Here's how the part is built. I have some questions about the finished solid (model axes, mm). Face numbers are marked on the shaded views. A direction names the side the tool comes from. Coordinates: 2 decimals unless noted, no trailing zeros. Order: outer loops, then holes, each group sorted by start corner. A loop starts at its lowest first (then second) coordinate and runs counter-clockwise, first axis right, second up. Notation, with made-up numbers: (71.5, -31) - (104.5, -31) arc R18 ccw to (104.5, -25) - close; hole circle Ø9 at (-16, 15.25). An arc over 180 degrees is marked (long way). Answer as CSV lines item,"result". Start each with the question number.
Item 1: Imagine slicing it at D-D on y = -2.5. List the corners of the cut face in (x, z) for me, and give its area (3 significant figures).
Item 2: We'd pull the mould along Y, two halves only. Please class the marked faces 1, 2 and 3: pulls with the +Y half, pulls with the -Y half, needs draft (parallel to the pull), parting line crosses it, or undercut.
Item 3: On a 3-axis mill with a long thin cutter (end or side, diameter ignored), from which of +Z, -Z, +X, -X, +Y, -Y can I reach the whole of each face in a straight line? I mean the marked faces 4, 5, 6 and 7. Say none if no direction works.
Item 4: I'm going to push flat-ended pins straight in: pin 1 (0.9 mm diameter, centred on y = 5.5, z = 2, fed in from +X); pin 2 (1.5 mm diameter, centred on y = 4, z = 1.5, fed in from -X); pin 3 (1.5 mm diameter, centred on x = -5.5, z = 1, fed in from -Y); pin 4 (4 mm diameter, centred on x = 2.5, y = 2.5, fed in from -Z). Where does each tip first touch, or does it pass through?
Item 5: Imagine slicing it at A-A on x = 5.5. List the corners of the cut face in (y, z) for me, and give its area (3 significant figures).
Item 6: I need wall thicknesses on line 1 (Y direction, x = -6, z = 2.5); line 2 (X direction, y = -0.25, z = 0.8); line 3 (Y direction, x = -3.5, z = 1.1). Which ranges of each line are inside material? Lowest first, please.
Item 7: Imagine slicing it at C-C on x = -5.5. List the corners of the cut face in (y, z) for me, and give its area (3 significant figures).
Item 8: Imagine slicing it at B-B on z = 0.25. List the corners of the cut face in (x, y) for me (3 decimals), and give its area (3 significant figures).
from build123d import *

# Parameters (mm, degrees)
SKETCH1_W           = 10.5
SKETCH1_H           = 22
BOSS_EXTRUDE1_DEPTH = 3
SKETCH2_W           = 6.75
SKETCH2_H           = 3
BOSS_EXTRUDE2_DEPTH = 3
SKETCH3_W           = 3
SKETCH3_H           = 3
BOSS_EXTRUDE3_DEPTH = 3
SKETCH4_W           = 2
SKETCH4_H           = 1.5
CUT_EXTRUDE1_DEPTH  = 3
SKETCH5_W           = 2
SKETCH5_H           = 10.5
CUT_EXTRUDE2_DEPTH  = 3
CHAMFER1_SIZE       = 0.25
CHAMFER2_SIZE       = 0.25
SKETCH6_W           = 3
SKETCH6_H           = 5
CUT_EXTRUDE3_DEPTH  = 0.5


with BuildPart() as part:
    # Sketch1 → Boss-Extrude1 (new body)
    with BuildSketch(Plane.XY):
        with Locations((1.5, 0)):
            Rectangle(SKETCH1_W, SKETCH1_H)
    extrude(amount=BOSS_EXTRUDE1_DEPTH)

    # Sketch2 → Boss-Extrude2 (add)
    with BuildSketch(Plane.XZ.offset(11)):
        with Locations((3, 1.5)):
            Rectangle(SKETCH2_W, SKETCH2_H)
    extrude(amount=BOSS_EXTRUDE2_DEPTH)

    # Sketch3 → Boss-Extrude3 (add)
    with BuildSketch(Plane.ZY.offset(3.75)):
        with Locations((1.5, -6.5)):
            Rectangle(SKETCH3_W, SKETCH3_H)
        with Locations((1.5, 6.5)):
            Rectangle(SKETCH3_W, SKETCH3_H)
    extrude(amount=BOSS_EXTRUDE3_DEPTH)

    # Sketch4 → Cut-Extrude1 (cut)
    with BuildSketch(Plane.XY.offset(3)):
        with Locations((5.75, -5.25)):
            Rectangle(SKETCH4_W, SKETCH4_H)
    extrude(amount=-CUT_EXTRUDE1_DEPTH, mode=Mode.SUBTRACT)

    # Sketch5 → Cut-Extrude2 (cut)
    with BuildSketch(Plane.XY.offset(3)):
        with Locations((5.75, 5.75)):
            Rectangle(SKETCH5_W, SKETCH5_H)
    extrude(amount=-CUT_EXTRUDE2_DEPTH, mode=Mode.SUBTRACT)

    # Chamfer1
    chamfer1_edges = [part.edges().sort_by_distance(p)[0] for p in [
        (4.75, -4.5, 1.5),
    ]]
    chamfer(chamfer1_edges, length=CHAMFER1_SIZE)

    # Chamfer2
    chamfer2_edges = [part.edges().sort_by_distance(p)[0] for p in [
        (4.75, -6, 1.5),
    ]]
    chamfer(chamfer2_edges, length=CHAMFER2_SIZE)

    # Sketch6 → Cut-Extrude3 (cut)
    with BuildSketch(Plane(origin=(6.75, 0, 0), x_dir=(0, 0, -1), z_dir=(1, 0, 0))):
        with Locations((-1.5, -2)):
            Rectangle(SKETCH6_W, SKETCH6_H)
    extrude(amount=-CUT_EXTRUDE3_DEPTH, mode=Mode.SUBTRACT)


solid = part.part
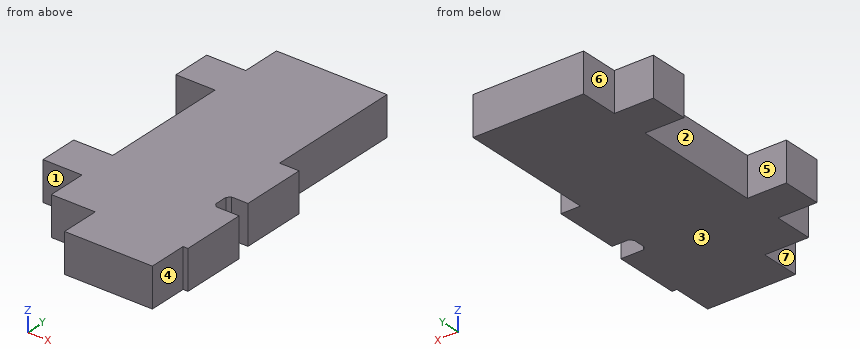
Responses:
1,outline,"(-3.75, 0) - (6.25, 0) - (6.25, 3) - (-3.75, 3) - close"
1,area,"30.0 mm^2"
2,face 1,"pulls with the -Y half"
2,face 2,"undercut"
2,face 3,"needs draft"
3,face 4,"+Z, -Z, +X, -Y"
3,face 5,"+Z, -Z, -X"
3,face 6,"+Z, -Z, -X, +Y"
3,face 7,"+Z, -Z, -X, -Y"
4,pin 1,"stops at x = 4.75"
4,pin 2,"stops at x = -3.75"
4,pin 3,"stops at y = -8"
4,pin 4,"stops at z = 0"
5,outline,"(-14, 0) - (-6, 0) - (-6, 3) - (-14, 3) - close; (-4.5, 0) - (0.5, 0) - (0.5, 3) - (-4.5, 3) - close"
5,area,"39.0 mm^2"
6,line 1,"y = -8 to -5, 5 to 8"
6,line 2,"x = -3.75 to 6.25"
6,line 3,"y = -11 to 11"
7,outline,"(-8, 0) - (-5, 0) - (-5, 3) - (-8, 3) - close; (5, 0) - (8, 0) - (8, 3) - (5, 3) - close"
7,area,"18.0 mm^2"
8,outline,"(-6.75, -8) - (-3.75, -8) - (-3.75, -11) - (-0.375, -11) - (-0.375, -14) - (6.375, -14) - (6.375, -11) - (6.75, -11) - (6.75, -6) - (5, -6) - (4.75, -5.75) - (4.75, -4.75) - (5, -4.5) - (6.25, -4.5) - (6.25, 0.5) - (4.75, 0.5) - (4.75, 11) - (-3.75, 11) - (-3.75, 8) - (-6.75, 8) - (-6.75, 5) - (-3.75, 5) - (-3.75, -5) - (-6.75, -5) - close"
8,area,"243 mm^2"
